from build123d import *

# Parameters (mm, degrees)
SKETCH1_R                                = 5
BOSS_EXTRUDE2_DEPTH                      = 109.22
CUT_EXTRUDE1_DEPTH                       = 2.54
TAP_DRILL_FOR_10_32_TAP1_D               = 4.0386
TAP_DRILL_FOR_10_32_TAP1_DEPTH           = 11.486682152
TAP_DRILL_FOR_10_32_TAP1_TIP             = 1.213317848
TAP_DRILL_FOR_10_32_TAP1_ON_FACE_2_D     = 4.0386
TAP_DRILL_FOR_10_32_TAP1_ON_FACE_2_DEPTH = 11.486682152
TAP_DRILL_FOR_10_32_TAP1_ON_FACE_2_TIP   = 1.213317848


with BuildPart() as part:
    # Sketch1 → Boss-Extrude2 (new body)
    with BuildSketch(Plane(origin=(0, 0, 0), x_dir=(1, 0, 0), z_dir=(0, 1, 0))):
        Circle(SKETCH1_R)
    extrude(amount=-BOSS_EXTRUDE2_DEPTH)

    # Sketch2 → Cut-Extrude1 (cut)
    with BuildSketch(Plane(origin=(0, 0, -5), x_dir=(-1, 0, 0), z_dir=(0, 0, -1))):
        with BuildLine():
            Line((-2, -109.22), (-2, -114.22))
            ThreePointArc((-2, -114.22), (0, -116.22), (2, -114.22))
            Line((2, -114.22), (2, -109.22))
            ThreePointArc((2, -109.22), (0, -107.22), (-2, -109.22))
        make_face()
        with BuildLine():
            Line((-1.5, -63.5), (-1.5, -68.5))
            ThreePointArc((-1.5, -68.5), (0, -70), (1.5, -68.5))
            Line((1.5, -68.5), (1.5, -63.5))
            ThreePointArc((1.5, -63.5), (0, -62), (-1.5, -63.5))
        make_face()
        with BuildLine():
            Line((-1.5, -10.39), (-1.5, -15.39))
            ThreePointArc((-1.5, -15.39), (0, -16.89), (1.5, -15.39))
            Line((1.5, -15.39), (1.5, -10.39))
            ThreePointArc((1.5, -10.39), (0, -8.89), (-1.5, -10.39))
        make_face()
    extrude(amount=-CUT_EXTRUDE1_DEPTH, mode=Mode.SUBTRACT)

    # Tap Drill for #10-32 Tap1
    with Locations(Plane.ZX):
        with Locations((0, 0)):
            Hole(TAP_DRILL_FOR_10_32_TAP1_D / 2, depth=TAP_DRILL_FOR_10_32_TAP1_DEPTH)
            with Locations((0, 0, -(TAP_DRILL_FOR_10_32_TAP1_DEPTH + TAP_DRILL_FOR_10_32_TAP1_TIP / 2))):  # 118° drill point
                Cone(0, TAP_DRILL_FOR_10_32_TAP1_D / 2, TAP_DRILL_FOR_10_32_TAP1_TIP, mode=Mode.SUBTRACT)

    # Tap Drill for #10-32 Tap1 on face 2
    with Locations(Plane(origin=(0, -109.22, 0), x_dir=(0, 0, -1), z_dir=(0, -1, 0))):
        with Locations((0, 0)):
            Hole(TAP_DRILL_FOR_10_32_TAP1_ON_FACE_2_D / 2, depth=TAP_DRILL_FOR_10_32_TAP1_ON_FACE_2_DEPTH)
            with Locations((0, 0, -(TAP_DRILL_FOR_10_32_TAP1_ON_FACE_2_DEPTH + TAP_DRILL_FOR_10_32_TAP1_ON_FACE_2_TIP / 2))):  # 118° drill point
                Cone(0, TAP_DRILL_FOR_10_32_TAP1_ON_FACE_2_D / 2, TAP_DRILL_FOR_10_32_TAP1_ON_FACE_2_TIP, mode=Mode.SUBTRACT)


solid = part.part
The listing builds one solid part. Answer for the finished solid, in the listing's coordinates (mm). A direction names the side the tool comes from. Give positions to 0.01 mm unless a question says otherwise; leave off trailing zeros. Write each loop counter-clockwise with the first axis right and the second up, starting at its lowest first coordinate (ties: lowest second). Pieces come first, ordered by that corner, then holes.
1) A tool of negligible diameter and unlimited length cuts with its end or side. For faces 5 (the face through (1.5, -66, -4)), 6 (the face through (-0.04, -107.22, -3.75)), 7 (the face through (0.607, -103.396, 1.926)), 8 (the face through (-0.34, -12.49, -0.08)), from which of +Z, -Z, +X, -X, +Y, -Y can it reach the whole face along a straight path? Write none if from no direction.
2) Find the intervals of material crossed by L1, parallel to Z at x = 0, y = -103; L2, parallel to Z at x = -0.25, y = -40.5, in increasing order.
3) For a pull along X with two mould halves and no side action, classify faces 1 (the face through (-1.08, -53.85, 4.88)), 2 (the face through (0, -70, -4)), 3 (the face through (-0.1, -109.22, 2.3)), 4 (the face through (-1.5, -66, -4)) as pulls with the +X half, pulls with the -X half, needs draft (parallel to the pull), parting line crosses it, or undercut.
4) Section B-B (y = -54.5) is taken. Write down the section's boundary in (x, z), and give its area (3 significant figures).
5) Section A-A (y = -102) is taken. Write down the section's boundary in (x, z).
6) Given P1, Ø1.2, axis at y = -65.5, z = -3.5, coming from the -X side; P2, Ø1, axis at y = -46, z = -3, coming from the +X side; P3, Ø2, axis at y = -48, z = -2, coming from the -X side, each flat-ended and moving along its own axis, determine where each tip first touches the part or whether it passes through.
7) Section C-C (x = 4) is taken. Write down the section's boundary in (y, z).
Response:
1. face 5: -Z
1. face 6: -Z, -Y
1. face 7: -Y
1. face 8: +Y
2. L1: z = -5 to -2.02, 2.02 to 5
2. L2: z = -4.99 to 4.99
3. face 1: parting line crosses it
3. face 2: undercut
3. face 3: needs draft
3. face 4: undercut
4. outline: circle Ø10 at (0, 0)
4. area: 78.5 mm2
5. outline: circle Ø10 at (0, 0); hole circle Ø4.04 at (0, 0)
6. P1: stops at x = -4.07
6. P2: stops at x = 4.33
6. P3: stops at x = -4.9
7. outline: (-109.22, -3) - (0, -3) - (0, 3) - (-109.22, 3) - close
